Input: part model. Units: mm. Frame: model coordinates. A direction names the side the tool comes from. Give positions to 0.01 mm unless a question says otherwise; leave off trailing zeros. Loops run counter-clockwise (first coordinate to the right, second up) from the corner with the lowest first, then second, coordinate; pieces in that order, holes last. Notation, with made-up numbers: (70.25, 69.25) -> (89.25, 69.25) arc R9 cw to (89.25, 84.25) -> close; hole circle Ø1 at (41, 79). An arc over 180 degrees is marked (long way). Answer as a JSON object with one key per item and string values.
```python
from build123d import *

# Parameters (mm, degrees)
F0_R     = 1.55
F1_DEPTH = 1.5
F2_R     = 2
F3_R     = 1


with BuildPart() as f1:
    # F0 (on Top) → F1 (new body)
    with BuildSketch(Plane.XY):
        Polygon((-14.33, 17.7), (-20.1, 17.7), (-20.1, -17.7), (-14.33, -17.7), (-14.33, -19.3), (-4.85, -19.3), (-4.85, -17.7), (0, -17.7), (4.85, -17.7), (4.85, -19.3), (14.33, -19.3), (14.33, -17.7), (20.1, -17.7), (20.1, 17.7), (14.33, 17.7), (14.33, 19.3), (4.85, 19.3), (4.85, 17.7), (0, 17.7), (-4.85, 17.7), (-4.85, 19.3), (-14.33, 19.3), align=None)
        with Locations((-14.25, -14)):
            Circle(F0_R, mode=Mode.SUBTRACT)
        with Locations((14.25, -14)):
            Circle(F0_R, mode=Mode.SUBTRACT)
        with Locations((-14.25, 14)):
            Circle(F0_R, mode=Mode.SUBTRACT)
        Polygon((-15.5, 9), (0, 13.5), (15.5, 9), (15.5, -9), (0, -13.5), (-15.5, -9), align=None, mode=Mode.SUBTRACT)
        with Locations((14.25, 14)):
            Circle(F0_R, mode=Mode.SUBTRACT)
    extrude(amount=F1_DEPTH)

    # F2
    f2_edges = [f1.edges().sort_by_distance(p)[0] for p in [
        (-15.5, -9, 0.75),
        (-15.5, 9, 0.75),
        (0, 13.5, 0.75),
        (15.5, 9, 0.75),
        (15.5, -9, 0.75),
        (0, -13.5, 0.75),
    ]]
    fillet(f2_edges, radius=F2_R)

    # F3
    f3_edges = [f1.edges().sort_by_distance(p)[0] for p in [
        (-20.1, 17.7, 0.75),
        (20.1, 17.7, 0.75),
        (20.1, -17.7, 0.75),
        (-20.1, -17.7, 0.75),
    ]]
    fillet(f3_edges, radius=F3_R)


solid = f1.part
```
Q1. Section A-A, the plane y = 14. Return the cut outline in (x, z).
Evaluation:
{"outline": "(-20.1, 0) -> (-15.8, 0) -> (-15.8, 1.5) -> (-20.1, 1.5) -> close; (-12.7, 0) -> (12.7, 0) -> (12.7, 1.5) -> (-12.7, 1.5) -> close; (15.8, 0) -> (20.1, 0) -> (20.1, 1.5) -> (15.8, 1.5) -> close"}
Q2. Pin query (flat end, axial travel): pin 1 (0.8 mm diameter, centred on x = -1, z = 1, fed in from -Y); pin 2 (0.8 mm diameter, centred on x = 2, z = 0.5, fed in from +Y). Return the tip coordinate at first contact, or that it passes through.
Evaluation:
{"pin 1": "stops at y = -17.7", "pin 2": "stops at y = 17.7"}
Q3. Section D-D, the plane z = 0.5. Give the number of separate pieces and of enclosed holes in the cut face, then the cut area to 3 significant figures.
Evaluation:
{"separate pieces": "1", "enclosed holes": "5", "area": "757 mm2"}
Q4. Section C-C, the plane x = 2.5. Return the cut outline in (y, z), then the cut area to 3 significant figures.
Evaluation:
{"outline": "(-17.7, 0) -> (-12.77, 0) -> (-12.77, 1.5) -> (-17.7, 1.5) -> close; (12.77, 0) -> (17.7, 0) -> (17.7, 1.5) -> (12.77, 1.5) -> close", "area": "14.8 mm2"}
Q5. Ray query, line 1 along Y through (x, z) = (-14.25, 0.45); line 2 along X through (y, z) = (2, 0.3); line 3 along Y through (x, z) = (13, 0.1). Return the intervals inside material, ascending.
Evaluation:
{"line 1": "y = -19.3 to -15.55, -12.45 to -9.35, 9.35 to 12.45, 15.55 to 19.3", "line 2": "x = -20.1 to -15.5, 15.5 to 20.1", "line 3": "y = -19.3 to -14.92, -13.08 to -9.73, 9.73 to 13.08, 14.92 to 19.3"}
Q6. Section B-B, the plane y = 1.5. Return the cut outline in (x, z), then the cut area to 3 significant figures.
Evaluation:
{"outline": "(-20.1, 0) -> (-15.5, 0) -> (-15.5, 1.5) -> (-20.1, 1.5) -> close; (15.5, 0) -> (20.1, 0) -> (20.1, 1.5) -> (15.5, 1.5) -> close", "area": "13.8 mm2"}
Q7. Draft query along Y for faces 1 (the flat face through (-10, 19.3, 1)), 2 (the flat face through (-7.213, -11.406, 0.74)), 3 (the flat face through (-14.33, 19, 1)), 4 (the flat face through (0, -17.7, 1)). Return one class per face: +Y half, -Y half, draft (parallel to the pull), parting line (faces both ways), or undercut.
Evaluation:
{"face 1": "+Y half", "face 2": "undercut", "face 3": "draft", "face 4": "-Y half"}
Q8. Access query for faces 5 (the cylindrical face through (-15.1, 8.7, 0.8)), 6 (the flat face through (14.33, -19, 1)), 7 (the flat face through (-17, 17.7, 1)), 8 (the flat face through (4.85, 19, 1)). Directions: +Z, -Z, +X, -X, +Y, -Y. A direction counts if a zero-diameter tool reaches every point of the face in a straight line with its end or side. Return the directions, or none.
Evaluation:
{"face 5": "+Z, -Z", "face 6": "+Z, -Z, +X, -Y", "face 7": "+Z, -Z, -X, +Y", "face 8": "+Z, -Z, +Y"}
